Could you check a few things on this model? Use its own coordinates, in mm. Face numbers are marked on the shaded views. A direction names the side the tool comes from. Give positions to 0.01 mm unless a question says otherwise; leave off trailing zeros. Loops run counter-clockwise (first coordinate to the right, second up) from the corner with the lowest first, then second, coordinate; pieces in that order, holes last. Notation, with made-up numbers: M 7.5,40.5 L 49.5,40.5 A34 ccw 49.5,74.5 Z; hole C 82,-6 d1. An arc over 180 degrees is marked long. Answer in a Markdown table with one row per item. Add a question column.
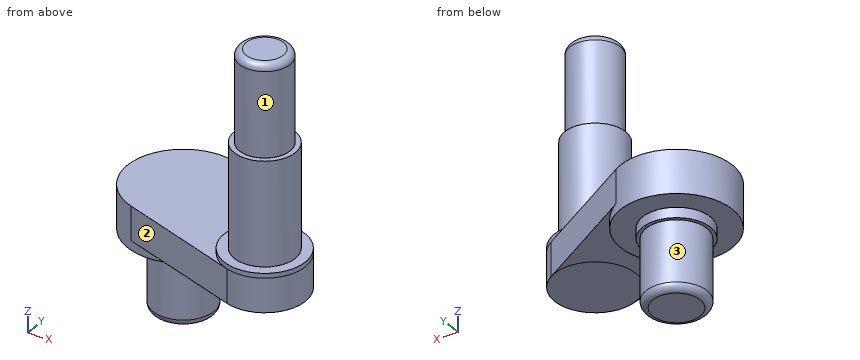
```python
from build123d import *
from build123d.topology import SkipClean

# Parameters (mm, degrees)
Y_KSEKLIK_EKSTR_ZYON1_DEPTH = 50
IZIM4_R                     = 60
Y_KSEKLIK_EKSTR_ZYON2_DEPTH = 57
IZIM5_R                     = 45
Y_KSEKLIK_EKSTR_ZYON3_DEPTH = 153
IZIM6_R                     = 37.5
Y_KSEKLIK_EKSTR_ZYON4_DEPTH = 135
RADYUS1_R                   = 10


with BuildPart() as part:
    # Çizim1 → Döndür1 (revolve)
    with BuildSketch(Plane(origin=(0, 0, 0), x_dir=(0, 0, -1), z_dir=(1, 0, 0)), mode=Mode.PRIVATE) as d_nd_r1_sk:
        with BuildLine():
            Line((0, 0), (100, 0))
            Line((100, 0), (100, 35))
            ThreePointArc((100, 35), (97.071067812, 42.071067812), (90, 45))
            Line((90, 45), (0, 45))
            Line((0, 45), (0, 0))
        make_face()
        Polygon((-15, 0), (0, 0), (0, 45), (0, 50), (-15, 50), align=None)
        Polygon((-79, 0), (-15, 0), (-15, 50), (-15, 82.5), (-79, 82.5), align=None)
    revolve(d_nd_r1_sk.sketch.rotate(Axis((0, 0, -100), (0, 0, 1)), 90), axis=Axis((0, 0, -100), (0, 0, 1)))

    # Çizim2 → Yükseklik-Ekstrüzyon1 (add)
    with BuildSketch(Plane.XY.offset(79)):
        with BuildLine():
            Line((204.064670252, -27.524722616), (42.86153958, 70.492116048))
            Line((42.86153958, 70.492116048), (-25.081375274, -78.595003749))
            Line((-25.081375274, -78.595003749), (154.651641268, -135.951718832))
            ThreePointArc((154.651641268, -135.951718832), (227.490317719, -103.673310664), (204.064670252, -27.524722616))
        make_face()
    extrude(amount=-Y_KSEKLIK_EKSTR_ZYON1_DEPTH)

    # Çizim4 → Yükseklik-Ekstrüzyon2 (add)
    with SkipClean():  # the faces are left unmerged after this step: merging them gives an invalid solid
        with BuildSketch(Plane(origin=(0, 0, 29), x_dir=(-1, 0, 0), z_dir=(0, 0, -1))):
            with Locations(Location((-172.892641467, -78.791716105, 0), (0, 0, 121.300985795))):
                Circle(IZIM4_R)
        extrude(amount=-Y_KSEKLIK_EKSTR_ZYON2_DEPTH)

    # Çizim5 → Yükseklik-Ekstrüzyon3 (add)
    with SkipClean():  # the faces are left unmerged after this step: merging them gives an invalid solid
        with BuildSketch(Plane.XY.offset(86)):
            with Locations((172.892641467, -78.791716105)):
                Circle(IZIM5_R)
        extrude(amount=Y_KSEKLIK_EKSTR_ZYON3_DEPTH)

    # Çizim6 → Yükseklik-Ekstrüzyon4 (add)
    with SkipClean():  # the faces are left unmerged after this step: merging them gives an invalid solid
        with BuildSketch(Plane.XY.offset(239)):
            with Locations((172.892641467, -78.791716105)):
                Circle(IZIM6_R)
        extrude(amount=Y_KSEKLIK_EKSTR_ZYON4_DEPTH)

    # Radyus1
    radyus1_edges = [part.edges().sort_by_distance(p)[0] for p in [
        (135.392641467, -78.791716105, 374),
    ]]
    fillet(radyus1_edges, radius=RADYUS1_R)


solid = part.part
```
Item 1: Suppose I cut it at D-D (y = 60.5). List the corners of the cut face in (x, z) for me.
Item 2: I need wall thicknesses on L1, parallel to Z at x = -67, y = 46.5; L2, parallel to Z at x = 39, y = 25; L3, parallel to Y at x = 3, z = -60.5. Which ranges of each line are inside material? Lowest first, please.
Item 3: Suppose I cut it at C-C (z = 97). List the corners of the cut face in (x, y) for me.
Item 4: Suppose I cut it at B-B (y = 0). List the corners of the cut face in (x, z) for me.
Item 5: For P1, Ø4, axis at x = 160.5, z = 70, coming from the +Y side; P2, Ø10, axis at x = 62, y = -104.5, coming from the -Z side; P3, Ø1, axis at x = 152, z = 215.5, coming from the -Y side, each with a flat end and sliding along its axis, tell me the tip position at first contact or that it passes through.
Item 6: For the marked faces 1, 2 and 3, which set-ups out of +Z, -Z, +X, -X, +Y, -Y let a thin tool reach every point of the face, with its end or its side?
Item 7: Suppose I cut it at A-A (x = 0). List the corners of the cut face in (y, z) for me, then the cut area to 3 significant figures.
Values found:
| question | item | result |
|---|---|---|
| 1 | outline | M -56.09,15 L 56.09,15 L 56.09,29 L 59.3,29 L 59.3,79 L -56.09,79 Z |
| 2 | L1 | 15 to 79 |
| 2 | L2 | 0 to 79 |
| 2 | L3 | -44.9 to 44.9 |
| 3 | outline | C 172.89,-78.79 d90 |
| 4 | outline | M -82.5,15 L -50,15 L -50,0 L -45,0 L -45,-90 A10 ccw -35,-100 L 35,-100 A10 ccw 45,-90 L 45,0 L 50,0 L 50,15 L 82.5,15 L 82.5,29 L 158.8,29 L 158.8,79 L -82.5,79 Z |
| 5 | P1 | y = 0.18 |
| 5 | P2 | z = 29 |
| 5 | P3 | y = -118.91 |
| 6 | face 1 | +Z |
| 6 | face 2 | +Z, -Z, -X, -Y |
| 6 | face 3 | -Z |
| 7 | outline | M -86.6,29 L -82.5,29 L -82.5,15 L -50,15 L -50,0 L -45,0 L -45,-90 A10 ccw -35,-100 L 35,-100 A10 ccw 45,-90 L 45,0 L 50,0 L 50,15 L 82.5,15 L 82.5,79 L -86.6,79 Z |
| 7 | area | 21,200 mm² |
